Source: three-view drawing plus pictorial views. Frame: mm from the lowest corner of the part. Give positions to 0.01 mm unless a question says otherwise; leave off trailing zeros. Order: outer loops, then holes, each group sorted by start corner. A loop starts at its lowest first (then second) coordinate and runs counter-clockwise, first axis right, second up. Notation, with made-up numbers: M 46,83.25 L 92,83.25 A25 ccw 92,116.25 Z; hole C -15,60 d11. An arc over 180 degrees is marked long. Use CSV: the item, a comma, the result in double quotes. Start each with the question number.
Item 1: Section query C-C on z = 1.8. Count the separate pieces of the cut face and the enclosed holes in it.
Item 2: Pull-direction query (Y, two-part tool) for the marked faces 1, 2 and 3; classes: +Y half, -Y half, draft (parallel to the pull), parting line (faces both ways), or undercut.
Item 3: Section query A-A on x = 10. Return loops of the section in (y, z).
Item 4: Ray query, probe 1 along Y at (x, z) = (10, 0.9); probe 2 along Y at (x, z) = (15.75, 1.15); probe 3 along X at (y, z) = (5.75, 0.7). Return the intervals inside material, ascending. Write a range as from..to.
Item 5: First-contact query: pin 1 (2 mm diameter, centred on x = 15.5, y = 2.5, fed in from -Z). Flat tip, straight axial feed; report the tip coordinate or a pass-through.
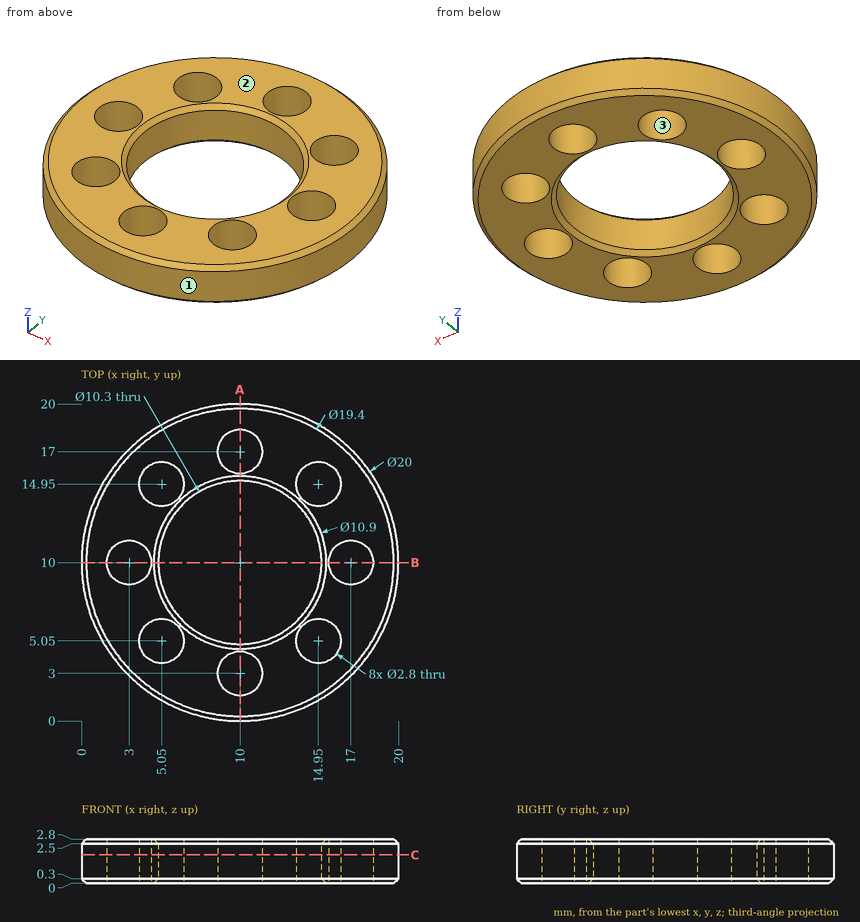
Verdict:
1,separate pieces,"1"
1,enclosed holes,"9"
2,face 1,"parting line"
2,face 2,"draft"
2,face 3,"undercut"
3,outline,"M 0,0.3 L 0.3,0 L 1.6,0 L 1.6,2.8 L 0.3,2.8 L 0,2.5 Z; M 4.4,0 L 4.55,0 L 4.85,0.3 L 4.85,2.5 L 4.55,2.8 L 4.4,2.8 Z; M 15.15,0.3 L 15.45,0 L 15.6,0 L 15.6,2.8 L 15.45,2.8 L 15.15,2.5 Z; M 18.4,0 L 19.7,0 L 20,0.3 L 20,2.5 L 19.7,2.8 L 18.4,2.8 Z"
4,probe 1,"0..1.6, 4.4..4.85, 15.15..15.6, 18.4..20"
4,probe 2,"1.82..3.9, 6.2..9.37, 10.63..13.8, 16.1..18.18"
4,probe 3,"0.95..3.84, 6.26..7.09, 12.91..13.74, 16.16..19.05"
5,pin 1,"z = 0"
